For this review, take the finished solid that the model builds, in its own axes (mm). A direction names the side the tool comes from. Give positions to 0.01 mm unless a question says otherwise; leave off trailing zeros. Write each loop counter-clockwise with the first axis right and the second up, starting at its lowest first coordinate (ties: lowest second). Pieces come first, ordered by that corner, then holes. Notation, with made-up numbers: (41.5, -39) -> (47.5, -39) arc R24 cw to (47.5, -29) -> close; hole circle Ø7 at (76.25, -8). An arc over 180 degrees is marked (long way). Answer as CSV lines item,"result".
```python
from build123d import *

# Parameters (mm, degrees)
DODANIE_WYCI_GNI_CIE1_DEPTH     = 14.25
ZAOKR_GLENIE1_R                 = 2
DODANIE_WYCI_GNI_CIE2_DEPTH     = 2
ZAOKR_GLENIE2_R                 = 1
ZAOKR_GLENIE3_R                 = 1
WYTNIJ_WYCI_GNI_CIE1_DEPTH      = 30.954621541
WYTNIJ_WYCI_GNI_CIE1_DEPTH_BACK = 30.954621541
SZKIC4_R                        = 1.225


with BuildPart() as part:
    # Szkic1 → Dodanie-wyciągnięcie1 (new body)
    with BuildSketch(Plane.XY):
        Polygon((1.783068787, -4.564092652), (-0.653727134, 7.430712848), (-12.25993137, 11.317788426), (-21.429339686, 3.210058505), (-18.992543765, -8.784746995), (-7.386339528, -12.671822573), align=None)
    extrude(amount=DODANIE_WYCI_GNI_CIE1_DEPTH)

    # Zaokrąglenie1
    zaokr_glenie1_edges = [part.edges().sort_by_distance(p)[0] for p in [
        (-7.386339528, -12.671822573, 7.125),
        (-18.992543765, -8.784746995, 7.125),
        (-21.429339686, 3.210058505, 7.125),
        (-12.25993137, 11.317788426, 7.125),
        (-0.653727134, 7.430712848, 7.125),
        (1.783068787, -4.564092652, 7.125),
    ]]
    fillet(zaokr_glenie1_edges, radius=ZAOKR_GLENIE1_R)

    # Szkic3 → Dodanie-wyciągnięcie2 (add)
    with BuildSketch(Plane.XY.offset(14.25)):
        Polygon((-0.091452095, 7.927884965), (-12.409357535, 12.053318952), (-22.141040889, 3.448416913), (-19.554818803, -9.281919113), (-7.236913363, -13.407353099), (2.494769991, -4.80245106), align=None)
    extrude(amount=-DODANIE_WYCI_GNI_CIE2_DEPTH)

    # Zaokrąglenie2
    zaokr_glenie2_edges = [part.edges().sort_by_distance(p)[0] for p in [
        (-6.456829252, 9.374250637, 0),
        (-2.80163537, -8.617957613, 0),
        (-13.189441647, -10.728284784, 0),
        (-20.210941725, -2.787344245, 0),
        (-16.844635528, 7.263923465, 0),
        (0.564670827, 1.433310098, 0),
        (-12.198333493, 11.014581025, 0),
        (-21.135955436, 3.111800131, 0),
        (-18.760757392, -8.579797968, 0),
        (-7.447937406, -12.368615173, 0),
        (1.489684537, -4.465834278, 0),
        (-0.885513507, 7.225763821, 0),
    ]]
    fillet(zaokr_glenie2_edges, radius=ZAOKR_GLENIE2_R)

    # Zaokrąglenie3
    zaokr_glenie3_edges = [part.edges().sort_by_distance(p)[0] for p in [
        (1.201658948, 1.562716953, 14.25),
        (-6.250404815, 9.990601959, 14.25),
        (-17.275199212, 7.750867932, 14.25),
        (-20.847929846, -2.9167511, 14.25),
        (-13.395866083, -11.344636106, 14.25),
        (-2.371071686, -9.10490208, 14.25),
    ]]
    fillet(zaokr_glenie3_edges, radius=ZAOKR_GLENIE3_R)

    # Szkic4 → Wytnij-wyciągnięcie1 (cut, two sides: drawn at the far end of the back side and taken through both)
    with BuildSketch(Plane(origin=(-0.257260592, 1.266331223, 0), x_dir=(0.9799817241599056, 0.19908746899937949, 0), z_dir=(-0.19908746899937946, 0.9799817241599055, 0)).offset(-WYTNIJ_WYCI_GNI_CIE1_DEPTH_BACK)):
        with Locations(Location((-9.76127883, -2.3, 0), (0, 0, 215.281261827))):
            Circle(SZKIC4_R)
    extrude(amount=WYTNIJ_WYCI_GNI_CIE1_DEPTH + WYTNIJ_WYCI_GNI_CIE1_DEPTH_BACK, mode=Mode.SUBTRACT)


solid = part.part
```
Q1. Draft analysis for pull direction Y (two halves, no side actions). For faces 1 (the cylindrical face through (-10.516, -0.988, 3.275)), 2 (the cylindrical face through (1.494, -4.452, 6.704)), 3 (the flat face through (-10, -1, 14.25)), state which applies: released by +Y, released by -Y, zero draft, split by the parting line, or undercut.
Answer block:
face 1,"undercut"
face 2,"split by the parting line"
face 3,"zero draft"
Q2. Add section A-A (z = 11.75). Write out the cut boundary in (x, y) (1 decimal).
Answer block:
outline,"(-21.2, 2.1) -> (-19.2, -7.7) arc R2 ccw to (-17.9, -9.2) -> (-8.5, -12.3) arc R2 ccw to (-6.5, -11.9) -> (0.9, -5.3) arc R2 ccw to (1.6, -3.4) -> (-0.4, 6.3) arc R2 ccw to (-1.7, 7.8) -> (-11.2, 11) arc R2 ccw to (-13.1, 10.6) -> (-20.6, 4) arc R2 ccw to start"
Q3. Add section B-B (z = 2.5). Write out the cut boundary in (x, y), plus the area to 3 significant figures.
Answer block:
outline,"(-21.2, 2.08) -> (-19.22, -7.65) arc R2 ccw to (-17.9, -9.15) -> (-8.71, -12.23) -> (-13.31, 10.39) -> (-20.56, 3.97) arc R2 ccw to start; (-10.94, 10.87) -> (-6.34, -11.75) -> (0.92, -5.33) arc R2 ccw to (1.55, -3.43) -> (-0.42, 6.3) arc R2 ccw to (-1.75, 7.8) -> close"
area,"331 mm2"
Q4. To check wall thickness, follow probe 1 along Z at (x, y) = (-8.25, -7.75); probe 2 along Z at (x, y) = (-9.5, 1.75); probe 3 along Y at (x, z) = (-8.5, 6). State the ranges of each line that lie inside material, in increasing order. Write a range as [from, to].
Answer block:
probe 1,"z = [0, 1.08], [3.52, 14.25]"
probe 2,"z = [0, 1.37], [3.23, 14.25]"
probe 3,"y = [-12.3, 10.06]"
Q5. For faces 4 (the cylindrical face through (-17.2, 7.5, 13.9)), 5 (the cylindrical face through (-21.13, 3.13, 6.7)), 6 (the flat face through (-13, -11, 12.25)), 7 (the cylindrical face through (-18.77, -8.57, 6.7)), list the 3-axis set-ups (+Z, -Z, +X, -X, +Y, -Y) from which the entire face can be reached by the end or side of a thin tool; tool diameter is ignored.
Answer block:
face 4,"+Z, -X, +Y"
face 5,"-Z, -X"
face 6,"-Z"
face 7,"-Z, -X, -Y"
Q6. Clearance check with flat-ended pins moving along their axes: pin 1 (6 mm diameter, centred on x = -0.5, z = 4.5, fed in from +Y); pin 2 (2 mm diameter, centred on x = -7.5, z = 4.5, fed in from -Y); pin 3 (5 mm diameter, centred on y = -6, z = 7, fed in from -X). State where each tip first meets the part, or that it passes through.
Answer block:
pin 1,"stops at y = 8.38"
pin 2,"stops at y = -12.41"
pin 3,"stops at x = -20.07"
